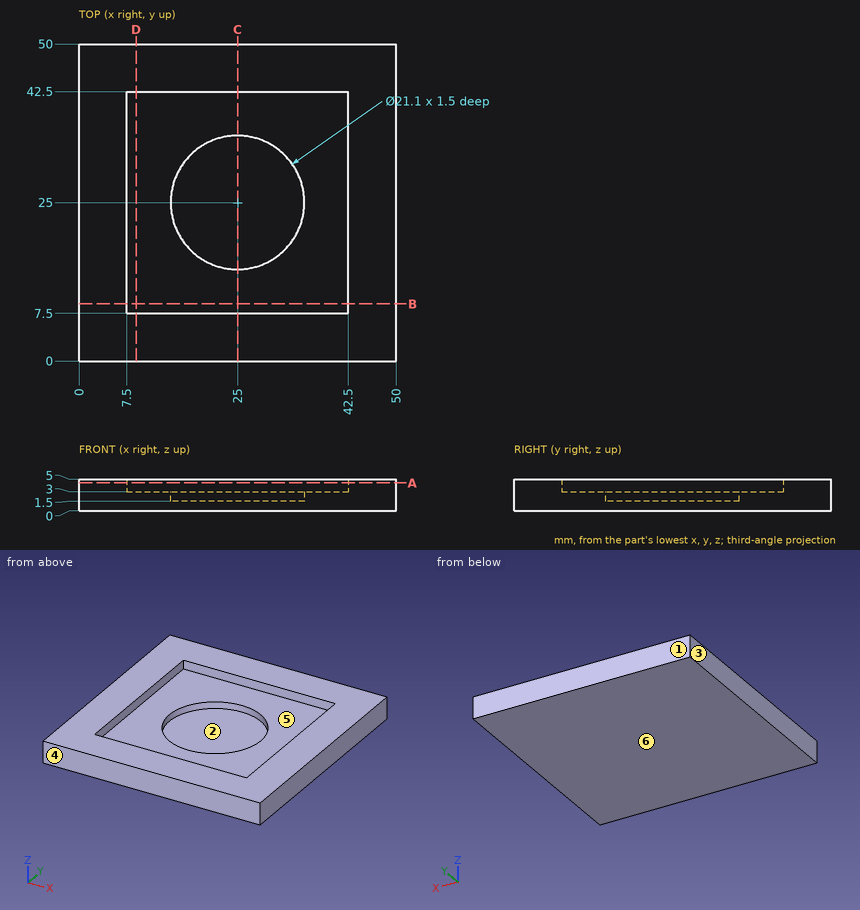
Check sheet for the drawn part. Datum: minimum x, y, z corner. Units: mm. A direction names the side the tool comes from. Coordinates: 2 decimals unless noted, no trailing zeros. Loops run counter-clockwise (first coordinate to the right, second up) from the corner with the lowest first, then second, coordinate; pieces in that order, holes last. Notation, with made-up numbers: (-26, 70) - (16, 70) arc R32 cw to (16, 103) - close; hole circle Ø3 at (-37.75, 16). An arc over 180 degrees is marked (long way). Put each result on its own line as item: value.
Item 1: Gauge pin test, flat ends, axial feed: pin 1 Ø19 at (x, y) = (25, 25) entering from +Z; pin 2 Ø17 at (x, y) = (23, 23.5) entering from +Z. Record the tip position at first contact, or that the pin passes through.
Conclusion:
pin 1: stops at z = 1.5
pin 2: stops at z = 3
Item 2: Set-up check for the marked faces 5 and 6: record each of +Z, -Z, +X, -X, +Y, -Y from which the full face is reachable in a straight line by a thin tool's end or side.
Conclusion:
face 5: +Z
face 6: -Z, +X, -X, +Y, -Y
Item 3: Section check A-A (z = 4.4). Enter the section's corners in (x, y).
Conclusion:
outline: (0, 0) - (50, 0) - (50, 50) - (0, 50) - close; hole (7.5, 7.5) - (42.5, 7.5) - (42.5, 42.5) - (7.5, 42.5) - close
Item 4: Scan lines: line 1 along Y through (x, z) = (25, 2.6); line 2 along Y through (x, z) = (41.5, 3.7). Record each from-to range of solid material in increasing order.
Conclusion:
line 1: y = 0 to 14.45, 35.55 to 50
line 2: y = 0 to 7.5, 42.5 to 50
Item 5: Section check B-B (y = 9). Enter the section's corners in (x, z), then the cut area to 3 significant figures.
Conclusion:
outline: (0, 0) - (50, 0) - (50, 5) - (42.5, 5) - (42.5, 3) - (7.5, 3) - (7.5, 5) - (0, 5) - close
area: 180 mm2
Item 6: Section check C-C (x = 25). Enter the section's corners in (y, z), then the cut area to 3 significant figures.
Conclusion:
outline: (0, 0) - (50, 0) - (50, 5) - (42.5, 5) - (42.5, 3) - (35.55, 3) - (35.55, 1.5) - (14.45, 1.5) - (14.45, 3) - (7.5, 3) - (7.5, 5) - (0, 5) - close
area: 148 mm2
Item 7: Draft check along Y on the marked faces 1, 2, 3 and 4. Enter one of: pulls with the +Y half, pulls with the -Y half, needs draft (parallel to the pull), parting line crosses it, or undercut.
Conclusion:
face 1: pulls with the +Y half
face 2: undercut
face 3: needs draft
face 4: pulls with the -Y half
